from build123d import *

# Parameters (mm, degrees)
F0_W          = 69.8839575052
F0_H          = 31.9469533861
F1_DEPTH      = 25.4
F3_DEPTH      = 31.9479533861
F5_DEPTH      = 5.08
F5_DEPTH_BACK = 36.83
F6_R          = 4.4661221371
F6_R_2        = 4.4516987215
F7_DEPTH      = 25.401


with BuildPart() as f1:
    # F0 (on Top) → F1 (new body)
    with BuildSketch(Plane.XY):
        with Locations((1.9966848195, 0.1426208764)):
            Rectangle(F0_W, F0_H)
    extrude(amount=F1_DEPTH)

    # F2 (on face) → F3 (cut, through all)
    with BuildSketch(Plane.XZ.offset(15.8308558166)):
        with BuildLine():
            Line((20.8225678653, 25.4), (-17.9701615125, 25.4))
            ThreePointArc((-17.9701615125, 25.4), (1.4262031764, 11.2350146431), (20.8225678653, 25.4))
        make_face()
    extrude(amount=-F3_DEPTH, mode=Mode.SUBTRACT)

    # F4 (on face) → F5 (join, two sides)
    with BuildSketch(Plane.XZ.offset(15.8308558166)) as f5_sk:
        with BuildLine():
            ThreePointArc((13.2335545495, 25.4485774785), (0.671350591, 16.2987194564), (-11.7973163724, 25.5756378174))
            Line((-11.7973163724, 25.5756378174), (-17.9701615125, 25.4))
            ThreePointArc((-17.9701615125, 25.4), (1.4262031764, 11.2350146431), (20.8225678653, 25.4))
            Line((20.8225678653, 25.4), (13.2335545495, 25.4485774785))
        make_face()
    extrude(amount=F5_DEPTH)
    extrude(f5_sk.sketch, amount=-F5_DEPTH_BACK)

    # F6 (on face) → F7 (cut, through all)
    with BuildSketch(Plane.XY.offset(25.4)):
        with Locations((-26.0657016188, 0)):
            Circle(F6_R)
        with Locations((29.4586159289, 0)):
            Circle(F6_R_2)
    extrude(amount=-F7_DEPTH, mode=Mode.SUBTRACT)


solid = f1.part
Here's how the part is built. I have some questions about the finished solid (model axes, mm). A direction names the side the tool comes from. Round coordinates to 2 decimals unless told otherwise and drop trailing zeros. Loops run counter-clockwise (first coordinate to the right, second up) from the corner with the lowest first, then second, coordinate; pieces in that order, holes last.
1. If we section it at D-D on x = -9.5: Write out the boundary of the cut face in (y, z).
Answer list:
outline: (-20.91, 14.41) - (-15.83, 14.41) - (-15.83, 0) - (16.12, 0) - (16.12, 14.41) - (21, 14.41) - (21, 21.22) - (-20.91, 21.22) - close
2. If we section it at B-B on z = 20: Write out the boundary of the cut face in (x, y).
Answer list:
outline: (-32.95, -15.83) - (-15.31, -15.83) - (-15.31, -20.91) - (-8.39, -20.91) - (-8.39, 21) - (-15.31, 21) - (-15.31, 16.12) - (-32.95, 16.12) - close; (9.87, -20.91) - (18.16, -20.91) - (18.16, -15.83) - (36.94, -15.83) - (36.94, 16.12) - (18.16, 16.12) - (18.16, 21) - (9.87, 21) - close; hole circle Ø8.93 at (-26.07, 0); hole circle Ø8.9 at (29.46, 0)
3. For P1, Ø7.5, axis at x = 8, z = 9, coming from the -Y side; P2, Ø10, axis at x = 0, z = 4, coming from the -Y side; P3, Ø17.5, axis at x = 32, y = -5, coming from the +Z side; P4, Ø7, axis at x = 29.46, y = 0, coming from the +Z side, each with a flat end and sliding along its axis, tell me the tip position at first contact or that it passes through.
Answer list:
P1: stops at y = -20.91
P2: stops at y = -15.83
P3: stops at z = 25.4
P4: passes through
4. If I drill on line 1 along X through (y, z) = (3.5, 24.25); line 2 along X through (y, z) = (-4, 11.75); line 3 along X through (y, z) = (-1, 3), over which ranges is the centre line in solid material (lowest first)?
Answer list:
line 1: x = -32.95 to -28.84, -23.29 to -11.31, 12.79 to 26.71, 32.21 to 36.94
line 2: x = -32.95 to -28.05, -24.08 to 27.5, 31.41 to 36.94
line 3: x = -32.95 to -30.42, -21.71 to 25.12, 33.8 to 36.94
5. We'd pull the mould along Y, two halves only. Please class faces 1 (the face through (2, 0, 0)), 2 (the face through (-30.528, 0.196, 12.878)), 3 (the face through (1, 20.999, 15)): +Y half, -Y half, draft (parallel to the pull), parting line (faces both ways), or undercut.
Answer list:
face 1: draft
face 2: undercut
face 3: +Y half
6. If we section it at C-C on y = 10: Write out the boundary of the cut face in (x, z).
Answer list:
outline: (-32.95, 0) - (36.94, 0) - (36.94, 25.4) - (20.82, 25.4) - (13.23, 25.45) arc R13.11 cw to (-11.8, 25.58) - (-17.97, 25.4) - (-32.95, 25.4) - close
7. Which directions (+Z, -Z, +X, -X, +Y, -Y) give clear straight access to the entire face, cutting with the end or side of a thin tool? Please do faces 4 (the face through (27, 4, 25.4)), 5 (the face through (1, -20.911, 15)), 6 (the face through (1.07, 18.52, 11.24)), 7 (the face through (2, -15.831, 10)), 8 (the face through (-22, 4, 25.4)).
Answer list:
face 4: +Z, +X, +Y, -Y
face 5: +Z, -Z, +X, -X, -Y
face 6: -Z, +Y
face 7: -Z, -Y
face 8: +Z, -X, +Y, -Y
8. If we section it at A-A on y = 0: Write out the boundary of the cut face in (x, z).
Answer list:
outline: (-32.95, 0) - (-30.53, 0) - (-30.53, 25.4) - (-32.95, 25.4) - close; (-21.6, 0) - (25.01, 0) - (25.01, 25.4) - (20.82, 25.4) - (13.23, 25.45) arc R13.11 cw to (-11.8, 25.58) - (-17.97, 25.4) - (-21.6, 25.4) - close; (33.91, 0) - (36.94, 0) - (36.94, 25.4) - (33.91, 25.4) - close
